```python
from build123d import *

# Parameters (mm, degrees)
BOSS_EXTRUDE1_DEPTH = 10
SKETCH2_R           = 1.5
BOSS_EXTRUDE2_DEPTH = 5
SKETCH3_W           = 4
SKETCH3_H           = 8
BOSS_EXTRUDE3_DEPTH = 12
SKETCH4_R           = 1
CUT_EXTRUDE1_DEPTH  = 38.725985739


with BuildPart() as part:
    # Sketch1 → Boss-Extrude1 (new body)
    with BuildSketch(Plane(origin=(0, 0, 0), x_dir=(0, 1, 0), z_dir=(0, 0, 1))):
        with BuildLine():
            Line((-13.5, 22), (13.5, 22))
            ThreePointArc((13.5, 22), (14.207106781, 21.707106781), (14.5, 21))
            Line((14.5, 21), (14.5, -21))
            ThreePointArc((14.5, -21), (14.207106781, -21.707106781), (13.5, -22))
            Line((13.5, -22), (-13.5, -22))
            ThreePointArc((-13.5, -22), (-14.207106781, -21.707106781), (-14.5, -21))
            Line((-14.5, -21), (-14.5, 21))
            ThreePointArc((-14.5, 21), (-14.207106781, 21.707106781), (-13.5, 22))
        make_face()
    extrude(amount=BOSS_EXTRUDE1_DEPTH)

    # Sketch2 → Boss-Extrude2 (add)
    with BuildSketch(Plane(origin=(-22, 0, 0), x_dir=(0, -1, 0), z_dir=(-1, 0, 0))):
        with Locations(Location((-12.5, 3, 0), (0, 0, 228.189685104))):
            Circle(SKETCH2_R)
        with Locations(Location((0.5, 3, 0), (0, 0, 270))):
            Circle(SKETCH2_R)
        with Locations(Location((6.5, 3, 0), (0, 0, 270))):
            Circle(SKETCH2_R)
        with Locations(Location((11.5, 3, 0), (0, 0, 270))):
            Circle(SKETCH2_R)
    extrude(amount=BOSS_EXTRUDE2_DEPTH)

    # Sketch3 → Boss-Extrude3 (add)
    with BuildSketch(Plane.XY.offset(10)):
        with Locations((-7, -9.5)):
            Rectangle(SKETCH3_W, SKETCH3_H)
        with Locations((-20, -9.5)):
            Rectangle(SKETCH3_W, SKETCH3_H)
    extrude(amount=BOSS_EXTRUDE3_DEPTH)

    # Sketch4 → Cut-Extrude1 (cut, through all)
    with BuildSketch(Plane(origin=(0, 0, 0), x_dir=(1, 0, 0), z_dir=(0, 0, -1))):
        with Locations(Location((-15, 12.5, 0), (0, 0, 180))):
            Circle(SKETCH4_R)
        with Locations(Location((15, 12.5, 0), (0, 0, 180))):
            Circle(SKETCH4_R)
        with Locations(Location((15, -12.5, 0), (0, 0, 180))):
            Circle(SKETCH4_R)
        with Locations(Location((-15, -12.5, 0), (0, 0, 180))):
            Circle(SKETCH4_R)
    extrude(amount=-CUT_EXTRUDE1_DEPTH, mode=Mode.SUBTRACT)


solid = part.part
```
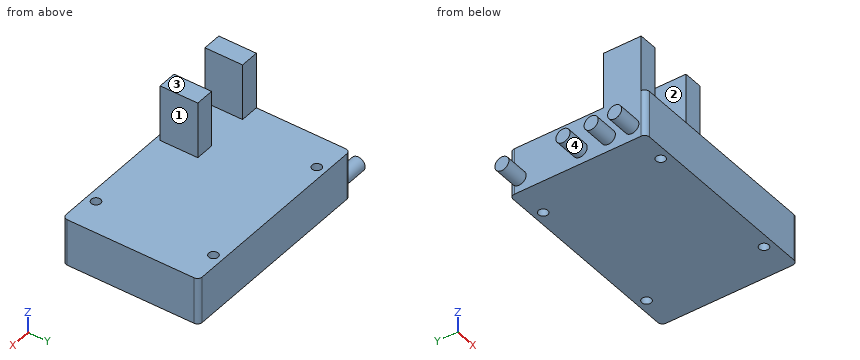
Geometry: final body of the model. Coordinates: model frame, mm. Face numbers are marked on the shaded views. A direction names the side the tool comes from. Round coordinates to 2 decimals unless told otherwise and drop trailing zeros. Order: outer loops, then holes, each group sorted by start corner. A loop starts at its lowest first (then second) coordinate and runs counter-clockwise, first axis right, second up. Notation, with made-up numbers: M 24,53.25 L 50,53.25 A16 cw 50,67.25 Z; hole C 74,38.5 d11. An arc over 180 degrees is marked long. One line per item, written item: value.
(1) Cut plane D-D (y = -6.5). Return the cut outline in (x, z).
Result sheet:
outline: M -27,1.5 L -22,1.5 L -22,0 L 22,0 L 22,10 L -5,10 L -5,22 L -9,22 L -9,10 L -18,10 L -18,22 L -22,22 L -22,4.5 L -27,4.5 Z
(2) Line query: probe 1 along Y at (x, z) = (-15, 4.5); probe 2 along X at (y, z) = (-12, 4); probe 3 along X at (y, z) = (-12.5, 16.5). Output: solid intervals per line, ascending. Write a range as [from, to].
Result sheet:
probe 1: [-14.5, -13.5], [-11.5, 11.5], [13.5, 14.5]
probe 2: [-27, -15.87], [-14.13, 14.13], [15.87, 22]
probe 3: [-22, -18], [-9, -5]
(3) Cut plane C-C (y = 12.5). Return the cut outline in (x, z).
Result sheet:
outline: M -27,1.5 L -22,1.5 L -22,0 L -16,0 L -16,10 L -22,10 L -22,4.5 L -27,4.5 Z; M -14,0 L 14,0 L 14,10 L -14,10 Z; M 16,0 L 22,0 L 22,10 L 16,10 Z
(4) Cut plane A-A (z = 19). Return the cut outline in (x, y).
Result sheet:
outline: M -22,-13.5 L -18,-13.5 L -18,-5.5 L -22,-5.5 Z; M -9,-13.5 L -5,-13.5 L -5,-5.5 L -9,-5.5 Z
(5) Pin query (flat end, axial travel): P1, Ø1.2, axis at x = -15, y = 12.5, coming from the +Z side; P2, Ø4, axis at y = -9.5, z = 16.5, coming from the +X side; P3, Ø2.5, axis at x = -15, y = -12.5, coming from the +Z side; P4, Ø4.5, axis at x = -20, z = 14, coming from the -Y side. Return the tip coordinate at first contact, or that it passes through.
Result sheet:
P1: through
P2: x = -5
P3: z = 10
P4: y = -13.5
(6) Cut plane B-B (x = -15). Return the cut outline in (y, z), and give its area (3 significant figures).
Result sheet:
outline: M -14.5,0 L -13.5,0 L -13.5,10 L -14.5,10 Z; M -11.5,0 L 11.5,0 L 11.5,10 L -11.5,10 Z; M 13.5,0 L 14.5,0 L 14.5,10 L 13.5,10 Z
area: 250 mm2
(7) Reachability of the marked faces 1, 2, 3 and 4 from +Z, -Z, +X, -X, +Y, -Y: full face, straight path, thin tool, end or side. Return the list, or none.
Result sheet:
face 1: +Z, +X, +Y, -Y
face 2: +Z, +Y, -Y
face 3: +Z, +X, -X, +Y, -Y
face 4: -X
